Part model, mm, in its own coordinate system. A direction names the side the tool comes from. Coordinates: 2 decimals unless noted, no trailing zeros. Write each loop counter-clockwise with the first axis right and the second up, starting at its lowest first coordinate (ties: lowest second). Pieces come first, ordered by that corner, then holes. Notation, with made-up numbers: (-13.75, -4.5) -> (-1.75, -4.5) arc R31 cw to (-1.75, 28.5) -> close; hole circle Ø5 at (-3.75, 76). An arc over 180 degrees is marked (long way). One line per question, with ' | ' between items. Start each with the question number.
Item 1: 3-axis set-ups, long thin cutter, end or side, ignore diameter. For faces 5 (the flat face through (3.25, 28.5, 10.1)), 6 (the cylindrical face through (-3.59, -5.6, 11.03)), 7 (the flat face through (3, -3.97, 8.6)): which of +Z, -Z, +X, -X, +Y, -Y reach the whole face in a straight line?
Item 2: Probe probe 1 along Y at (x, z) = (7.5, 10); probe 2 along Z at (x, y) = (6, 25); probe 3 along Y at (x, z) = (-4.5, 10). List the from-to ranges inside material, lowest first. Write a range as [from, to].
Item 3: Saw through at B-B (x = 0). List the corners of the cut face in (y, z), and give its area (3 significant figures).
Item 4: Saw through at A-A (y = 25). List the corners of the cut face in (x, z), and give its area (3 significant figures).
Item 5: Pin check, flat tips, straight feed: pin 1 (4 mm diameter, centred on y = -4.651, z = 10, fed in from -X); pin 2 (3 mm diameter, centred on y = 6, z = 10, fed in from +X); pin 3 (6.5 mm diameter, centred on x = -20.15, z = 10, fed in from +Y). Stop position of each tip, or through.
Item 6: Two-plate mould, pull along X, no slides. Class faces 1 (the flat face through (10, 12, 8)), 2 (the flat face through (-30, 32, 10)), 3 (the flat face through (0, 27.471, 10)), 4 (the flat face through (-10, 35, 10)): pulls with the +X half, pulls with the -X half, needs draft (parallel to the pull), parting line crosses it, or undercut.
Item 7: Saw through at D-D (z = 10). Count the separate pieces of the cut face and the enclosed holes in it, and give its area (3 significant figures).
Item 8: Saw through at C-C (z = 5.5). List the corners of the cut face in (x, y), and give its area (3 significant figures).
Autodesk Inventor part; units mm, degrees
ref_plane "Work Plane2" through (-30, -220, 20) normal (0, 0, 1) x (1, 0, 0)
ref_plane "YZ Plane" through (0, 0, 0) normal (1, 0, 0) x (0, 1, 0)
ref_plane "XZ Plane" through (0, 0, 0) normal (0, 1, 0) x (-1, 0, 0)
ref_plane "Work Plane1" through (0, 0, 0) normal (0, 0, 1) x (1, 0, 0)
sketch "Sketch1" plane through (0, 0, 0) normal (0, 0, 1) x (1, 0, 0)
  circle A0 centre (0, 0) radius 2 construction
  circle A1 centre (0, 20) radius 2.5 construction
  line L0 (-10, 4) -> (-10, 16) construction
  line L1 (-10, 4) -> (-6, 4) construction
  line L2 (-6, 4) -> (-6, -4) construction
  line L3 (-6, -4) -> (-10, -4) construction
  line L4 (-10, -4) -> (-10, -10) construction
  line L5 (-10, -10) -> (-4, -10) construction
  line L6 (-4, -10) -> (-4, -6) construction
  line L7 (-4, -6) -> (4, -6) construction
  line L8 (4, -6) -> (4, -10) construction
  line L9 (4, -10) -> (10, -10) construction
  line L10 (10, -10) -> (10, -4) construction
  line L11 (10, -4) -> (6, -4) construction
  line L12 (6, -4) -> (6, 4) construction
  line L13 (6, 4) -> (10, 4) construction
  line L14 (10, 4) -> (10, 16) construction
  line L15 (6, 16) -> (10, 16) construction
  line L16 (6, 24) -> (6, 16) construction
  line L17 (10, 24) -> (6, 24) construction
  line L18 (10, 30) -> (10, 24) construction
  line L19 (4, 30) -> (10, 30) construction
  line L20 (4, 26) -> (4, 30) construction
  line L21 (-4, 26) -> (4, 26) construction
  line L22 (-4, 30) -> (-4, 26) construction
  line L23 (-10, 30) -> (-4, 30) construction
  line L24 (-10, 24) -> (-10, 30) construction
  line L25 (-6, 24) -> (-10, 24) construction
  line L26 (-6, 16) -> (-6, 24) construction
  line L27 (-10, 16) -> (-6, 16) construction
  line L28 (-4, 6) -> (-4, 14) construction
  line L29 (4, 14) -> (-4, 14) construction
  line L30 (4, 6) -> (4, 14) construction
  line L31 (4, 6) -> (-4, 6) construction
  line L32 (10, 30) -> (-10, 30)
  line L33 (-10, 30) -> (-10, -10)
  line L34 (-10, -10) -> (10, -10)
  line L35 (10, -10) -> (10, 30)
  circle A2 centre (0, 20) radius 2.5
  circle A3 centre (0, 0) radius 2.5
  point P0 (0, 0)
  dimension "d0" = 40
  dimension "d1" = 5
ref_plane "Work Plane2" through (-30, -220, 20) normal (0, 0, 1) x (1, 0, 0)
extrude "Extrusion1" add sketch "Sketch1" along normal up to surface (20 mm away)
sketch "Sketch2" plane through (10, -10, 0) normal (1, 0, 0) x (0, 0, -1)
  line L0 (-20, 40) -> (-20, 0)
  line L1 (0, 0) -> (-20, 0)
  line L2 (0, 0) -> (0, 40)
  line L3 (0, 40) -> (-20, 40)
  line L4 (-14, 40) -> (-14, -210)
  line L5 (-6, 40) -> (-6, -210)
  line L6 (-20, 32.5) -> (-20, 27.5)
  line L7 (0, 32.5) -> (0, 27.5)
  line L8 (-20, 12.5) -> (-20, 7.5)
  line L9 (0, 12.5) -> (-20, 12.5)
  line L10 (0, 7.5) -> (-20, 7.5)
  line L11 (0, 32.5) -> (-20, 32.5)
  line L12 (0, 27.5) -> (-20, 27.5)
  circle A0 centre (-10, 45) radius 1.4
  circle A1 centre (-10, 25.349) radius 1.4
  circle A2 centre (-10, 15.349) radius 1.4
  circle A3 centre (-10, 35) radius 1.4
  circle A4 centre (-10, 5.349) radius 1.4
  point P0 (0, 10)
  point P1 (-9.8573, 5.349)
  dimension "d5" = 2.8
  dimension "d8" = 10
  dimension "d13" = 2.8
  dimension "d14" = 10
hole "Hole1" at (10, 25, 10) at (10, 5.349, 10) at (10, -4.651, 10) at (10, 15.349, 10) direction (-1, 0, 0) diameter 2.8 end through all counterbore diameter 6.5 counterbore depth 7
sketch "Sketch3" plane through (-10, 30, 0) normal (0, 1, 0) x (1, 0, 0)
  line L0 (0, -20) -> (20, -20)
  line L1 (20, 0) -> (20, -20)
  line L2 (20, 0) -> (0, 0)
  line L3 (0, 0) -> (0, -20)
  line L4 (20, 0) -> (0, 0)
  line L5 (20, 0) -> (-20, 0)
  line L6 (-20, 0) -> (-20, -20)
  line L7 (-20, -20) -> (20, -20)
  line L8 (20, -20) -> (20, 0)
  circle A0 centre (-10.1547, -10) radius 2.5
  point P0 (10, 0)
  dimension "d22" = 40
  dimension "d23" = 5
extrude "Extrusion2" add sketch "Sketch3" along normal blind 5
sketch "Sketch5" plane through (-10, -10, 20) normal (0, 0, 1) x (1, 0, 0)
  line L0 (6.75, 39.4711) -> (13.25, 39.4711)
  line L1 (13.25, 39.4711) -> (13.25, 37.4711)
  line L2 (13.25, 37.4711) -> (6.75, 37.4711)
  line L3 (6.75, 37.4711) -> (6.75, 39.4711)
  line L4 (6.75, 39.4711) -> (13.25, 37.4711) construction
  line L5 (13.25, 39.4711) -> (6.75, 37.4711) construction
  point P0 (10, 10)
  point P1 (10, 38.4711)
  dimension "d33" = 6.5
  dimension "d34" = 2
extrude "Extrusion3" cut sketch "Sketch5" against normal through all
properties part number "Neje_20mm_rod_connector_double"
From the geometry:
1) face 5: +Z, -Z | face 6: +X, -X | face 7: +X
2) probe 1: [-10, -7.9], [-1.4, 2.1], [8.6, 12.1], [18.6, 21.75], [28.25, 35] | probe 2: [0, 6.75], [13.25, 20] | probe 3: [-10, -6.05], [-3.25, 3.95], [6.75, 13.95], [16.75, 23.6], [26.4, 35]
3) outline: (-10, 0) -> (-2.5, 0) -> (-2.5, 20) -> (-10, 20) -> close; (2.5, 0) -> (17.5, 0) -> (17.5, 20) -> (2.5, 20) -> close; (22.5, 0) -> (27.47, 0) -> (27.47, 20) -> (22.5, 20) -> close; (29.47, 0) -> (35, 0) -> (35, 20) -> (29.47, 20) -> close; hole circle Ø2.8 at (-4.65, 10); hole circle Ø2.8 at (5.35, 10); hole circle Ø2.8 at (15.35, 10); hole circle Ø2.8 at (25, 10) | area: 635 mm2
4) outline: (-10, 0) -> (10, 0) -> (10, 6.75) -> (3, 6.75) -> (3, 8.6) -> (-10, 8.6) -> close; (-10, 11.4) -> (3, 11.4) -> (3, 13.25) -> (10, 13.25) -> (10, 20) -> (-10, 20) -> close | area: 318 mm2
5) pin 1: x = -10 | pin 2: x = 3 | pin 3: y = 35
6) face 1: pulls with the +X half | face 2: pulls with the -X half | face 3: undercut | face 4: needs draft
7) separate pieces: 6 | enclosed holes: 2 | area: 595 mm2
8) outline: (-30, 30) -> (-10, 30) -> (-10, -10) -> (10, -10) -> (10, 35) -> (-30, 35) -> close; hole (-3.25, 27.47) -> (3.25, 27.47) -> (3.25, 29.47) -> (-3.25, 29.47) -> close; hole circle Ø5 at (0, 0); hole circle Ø5 at (0, 20) | area: 948 mm2
